from build123d import *

# Parameters (mm, degrees)
SKETCH1_R           = 2.4892
BOSS_EXTRUDE1_DEPTH = 3.175
FILLET2_R           = 8.89
CUT_EXTRUDE2_DEPTH  = 246.195529119
FILLET3_R           = 1.5875


with BuildPart() as part:
    # Sketch1 → Boss-Extrude1 (new, symmetric)
    with BuildSketch(Plane(origin=(0, 0, 0), x_dir=(1, 0, 0), z_dir=(0, 1, 0))):
        Polygon((139.7, 25.4), (139.7, 107.95), (50.8, 107.95), (50.8, 146.05), (0, 146.05), (0, 107.95), (0, 44.45), (50.8, 44.45), (152.4, -53.975), (196.85, -53.975), (196.85, 0), (196.85, 25.4), align=None)
        with Locations(Location((184.15, -44.45, 0), (0, 0, 270))):
            Circle(SKETCH1_R, mode=Mode.SUBTRACT)
        with Locations(Location((184.15, 12.7, 0), (0, 0, 270))):
            Circle(SKETCH1_R, mode=Mode.SUBTRACT)
        with Locations(Location((12.7, 69.85, 0), (0, 0, 270))):
            Circle(SKETCH1_R, mode=Mode.SUBTRACT)
        with Locations(Location((12.7, 127, 0), (0, 0, 270))):
            Circle(SKETCH1_R, mode=Mode.SUBTRACT)
    extrude(amount=BOSS_EXTRUDE1_DEPTH, both=True)

    # Fillet2
    fillet2_edges = [part.edges().sort_by_distance(p)[0] for p in [
        (50.8, 0, -107.95),
        (139.7, 0, -107.95),
        (139.7, 0, -25.4),
        (196.85, 0, -25.4),
        (196.85, 0, 53.975),
        (152.4, 0, 53.975),
        (50.8, 0, -44.45),
        (0, 0, -44.45),
        (0, 0, -146.05),
        (50.8, 0, -146.05),
    ]]
    fillet(fillet2_edges, radius=FILLET2_R)

    # Sketch4 → Cut-Extrude2 (cut, through all)
    with BuildSketch(Plane(origin=(0, 3.175, 0), x_dir=(1, 0, 0), z_dir=(0, 1, 0))):
        with BuildLine():
            Line((32.261000835, 78.9647419), (52.342813318, 54.372399446))
            Line((52.342813318, 54.372399446), (72.424625802, 78.9647419))
            ThreePointArc((72.424625802, 78.9647419), (69.796699914, 95.436110561), (53.736462526, 90.93269463))
            Line((53.736462526, 90.93269463), (52.342813318, 88.079912324))
            Line((52.342813318, 88.079912324), (50.949164111, 90.93269463))
            ThreePointArc((50.949164111, 90.93269463), (34.888926723, 95.436110561), (32.261000835, 78.9647419))
        make_face()
        with BuildLine():
            Line((76.202071803, 36.3968294), (96.283884286, 11.804486946))
            Line((96.283884286, 11.804486946), (116.365696769, 36.3968294))
            ThreePointArc((116.365696769, 36.3968294), (113.737770882, 52.868198061), (97.677533493, 48.36478213))
            Line((97.677533493, 48.36478213), (96.283884286, 45.511999824))
            Line((96.283884286, 45.511999824), (94.890235079, 48.36478213))
            ThreePointArc((94.890235079, 48.36478213), (78.82999769, 52.868198061), (76.202071803, 36.3968294))
        make_face()
        with BuildLine():
            Line((120.14314277, -6.171083099), (140.224955253, -30.763425554))
            Line((140.224955253, -30.763425554), (160.306767736, -6.171083099))
            ThreePointArc((160.306767736, -6.171083099), (157.678841849, 10.300285561), (141.618604461, 5.796869631))
            Line((141.618604461, 5.796869631), (140.224955253, 2.944087324))
            Line((140.224955253, 2.944087324), (138.831306046, 5.796869631))
            ThreePointArc((138.831306046, 5.796869631), (122.771068658, 10.300285561), (120.14314277, -6.171083099))
        make_face()
    extrude(amount=-CUT_EXTRUDE2_DEPTH, mode=Mode.SUBTRACT)

    # Fillet3
    fillet3_edges = [part.edges().sort_by_distance(p)[0] for p in [
        (52.342813318, 0, -88.079912324),
        (52.342813318, 0, -54.372399446),
        (140.224955253, 0, -2.944087324),
        (140.224955253, 0, 30.763425554),
        (96.283884286, 0, -11.804486946),
        (96.283884286, 0, -45.511999824),
    ]]
    fillet(fillet3_edges, radius=FILLET3_R)


solid = part.part
The listing builds one solid part. Answer for the finished solid, in the listing's coordinates (mm). A direction names the side the tool comes from. Coordinates: 2 decimals unless noted, no trailing zeros. Write each loop counter-clockwise with the first axis right and the second up, starting at its lowest first coordinate (ties: lowest second). Pieces come first, ordered by that corner, then holes. Notation, with made-up numbers: (82.25, -4) -> (138.25, -4) arc R23 ccw to (138.25, 4) -> close; hole circle Ø6 at (5, 53.25). An arc over 180 degrees is marked (long way). One line per question, with ' | ' between items.
1. Which of the six approach directions +Z, -Z, +X, -X, +Y, -Y give full straight-line access (tool end or side, diameter ignored) to faces 4 (the cylindrical face through (2.54, 0.04, -143.38)), 5 (the flat face through (41.56, 0.04, -67.58)), 6 (the flat face through (50.8, 0, -127))?
Verdict:
face 4: -Z, -X, +Y, -Y | face 5: +Y, -Y | face 6: -Z, +X, +Y, -Y
2. Straight lines are drawn through the part: line 1 (X direction, y = -0.25, z = -9); line 2 (X direction, y = -2.5, z = -49.5); line 3 (X direction, y = 1, z = -124). For each, find the intervals that lie inside material, in ascending order.
Verdict:
line 1: x = 87.39 to 121.11, 136.48 to 143.97, 159.34 to 196.85 | line 2: x = 0.87 to 75.46, 94.25 to 98.32, 117.11 to 139.7 | line 3: x = 0 to 50.8
3. Section B-B (z = -127) is taken. Determine the outline of the cut face in (x, y) (3 decimals), and give its area (3 significant figures).
Verdict:
outline: (0, -3.175) -> (10.211, -3.175) -> (10.211, 3.175) -> (0, 3.175) -> close; (15.189, -3.175) -> (50.8, -3.175) -> (50.8, 3.175) -> (15.189, 3.175) -> close | area: 291 mm^2
4. Section A-A (x = 184.15) is taken. Determine the outline of the cut face in (y, z) (3 decimals).
Verdict:
outline: (-3.175, -25.4) -> (3.175, -25.4) -> (3.175, -15.189) -> (-3.175, -15.189) -> close; (-3.175, -10.211) -> (3.175, -10.211) -> (3.175, 41.961) -> (-3.175, 41.961) -> close; (-3.175, 46.939) -> (3.175, 46.939) -> (3.175, 53.975) -> (-3.175, 53.975) -> close
5. Section C-C (y = -1.5) is taken. State how many separate pieces and enclosed holes the cut face has, and give its area (3 significant figures).
Verdict:
separate pieces: 1 | enclosed holes: 7 | area: 15,400 mm^2
6. For a pull along Z with two mould halves and no side action, classify faces 1 (the flat face through (106.808, 0.044, -24.692)), 2 (the flat face through (119, -3.175, -47)), 3 (the flat face through (28, 0, -44.45)) as released by +Z, released by -Z, zero draft, split by the parting line, or undercut.
Verdict:
face 1: undercut | face 2: zero draft | face 3: released by +Z
7. Section D-D (z = -69.85) is taken. Determine the outline of the cut face in (x, y) (3 decimals).
Verdict:
outline: (0, -3.175) -> (10.211, -3.175) -> (10.211, 3.175) -> (0, 3.175) -> close; (15.189, -3.175) -> (39.704, -3.175) -> (39.704, 3.175) -> (15.189, 3.175) -> close; (64.982, -3.175) -> (139.7, -3.175) -> (139.7, 3.175) -> (64.982, 3.175) -> close
8. Given pin 1 Ø1.5 at (x, y) = (83.5, -1) entering from -Z; pin 2 Ø1.9 at (y, z) = (0, -52.5) entering from +X; pin 3 Ø1.5 at (y, z) = (-1.5, -3) entering from -X, each flat-ended and moving along its own axis, determine where each tip first touches the part or whether it passes through.
Verdict:
pin 1: stops at z = -107.95 | pin 2: stops at x = 139.7 | pin 3: stops at x = 92.81
